Source: CAD feature listing. Evaluate the final solid. Frame: model axes, mm. A direction names the side the tool comes from. Give positions to 0.01 mm unless a question says otherwise; leave off trailing zeros. Write each loop counter-clockwise with the first axis right and the second up, starting at its lowest first coordinate (ties: lowest second). Pieces come first, ordered by that corner, then holes. Notation, with made-up numbers: (-19.5, 18.5) - (27.5, 18.5) arc R23 ccw to (27.5, 33.5) - close; hole circle Ø2 at (75, 6). An arc over 180 degrees is marked (long way). One line per question, with ' | ' between items. Start each with the question number.
(1) Pin query (flat end, axial travel): pin 1 (5 mm diameter, centred on x = 12, z = 20.5, fed in from +Y); pin 2 (2.5 mm diameter, centred on y = -16, z = 33, fed in from -X); pin 3 (10 mm diameter, centred on x = 0, y = 0, fed in from +Z); pin 4 (12 mm diameter, centred on x = 18, y = 1.5, fed in from +Z). Return the tip coordinate at first contact, or that it passes through.
(2) Draft query along Y for faces 5 (the cylindrical face through (27, -16, 21)), 6 (the cylindrical face through (6.5, 0.07, 2.96)), 7 (the flat face through (0, -14.5, 21)). Return one class per face: +Y half, -Y half, draft (parallel to the pull), parting line (faces both ways), or undercut.
(3) Access query for faces 1 (the flat face through (17.5, 0, 3)), 2 (the flat face through (-17.5, 0, 3)), 3 (the flat face through (-17.5, -16, 33)), 4 (the flat face through (17.5, -16, 33)). Directions: +Z, -Z, +X, -X, +Y, -Y. A direction counts if a zero-diameter tool reaches every point of the face in a straight line with its end or side. Return the directions, or none.
(4) Ray query, line 1 (X direction, y = -16.4, z = 21); line 2 (Y direction, x = 0, z = 1.75); line 3 (Y direction, x = 8, z = 4.1). Return the intervals inside material, ascending. Write a range as [from, to].
(5) Section B-B, the plane y = 0. Return loops of the section in (x, z), plus the area to 3 significant figures.
(6) Section D-D, the plane z = 5. Return loops of the section in (x, y), plus the area to 3 significant figures.
(7) Section A-A, the plane x = 0. Return loops of the section in (y, z).
(8) Section C-C, the plane z = 21. Return loops of the section in (x, y), plus the area to 3 significant figures.
```python
from build123d import *

# Parameters (mm, degrees)
SKETCH1_W           = 35
SKETCH1_H           = 35
SKETCH1_R           = 5.5
SKETCH1_R_2         = 1.5
BOSS_EXTRUDE1_DEPTH = 6
SKETCH2_W           = 35
SKETCH2_H           = 3
BOSS_EXTRUDE2_DEPTH = 30
SKETCH3_R           = 1.5
BOSS_EXTRUDE3_DEPTH = 3


with BuildPart() as part:
    # Sketch1 → Boss-Extrude1 (new body)
    with BuildSketch(Plane.XY):
        Rectangle(SKETCH1_W, SKETCH1_H)
        Circle(SKETCH1_R, mode=Mode.SUBTRACT)
        with Locations((8, 0)):
            Circle(SKETCH1_R_2, mode=Mode.SUBTRACT)
        with Locations((-8, 0)):
            Circle(SKETCH1_R_2, mode=Mode.SUBTRACT)
    extrude(amount=BOSS_EXTRUDE1_DEPTH)

    # Sketch2 → Boss-Extrude2 (add)
    with BuildSketch(Plane.XY.offset(6)):
        with Locations((0, -16)):
            Rectangle(SKETCH2_W, SKETCH2_H)
    extrude(amount=BOSS_EXTRUDE2_DEPTH)

    # Sketch3 → Boss-Extrude3 (add)
    # profile 1 of 2: a face of its own
    with BuildSketch(Plane(origin=(0, -14.5, 0), x_dir=(1, 0, 0), z_dir=(0, 1, 0))):
        with BuildLine():
            Line((17.5, -29.75), (17.5, -12.25))
            Line((17.5, -12.25), (26.114080353, -19.090878575))
            ThreePointArc((26.114080353, -19.090878575), (27, -21), (26.114080353, -22.909121425))
            Line((26.114080353, -22.909121425), (17.5, -29.75))
        make_face()
        with Locations(Location((24.5, -21, 0), (0, 0, 270))):
            Circle(SKETCH3_R, mode=Mode.SUBTRACT)
    # profile 2 of 2: a face of its own
    with BuildSketch(Plane(origin=(0, -14.5, 0), x_dir=(1, 0, 0), z_dir=(0, 1, 0))):
        with BuildLine():
            Line((-17.5, -29.75), (-17.5, -12.25))
            Line((-17.5, -12.25), (-26.114080353, -19.090878575))
            ThreePointArc((-26.114080353, -19.090878575), (-27, -21), (-26.114080353, -22.909121425))
            Line((-26.114080353, -22.909121425), (-17.5, -29.75))
        make_face()
        with Locations(Location((-24.5, -21, 0), (0, 0, 270))):
            Circle(SKETCH3_R, mode=Mode.SUBTRACT)
    extrude(amount=-BOSS_EXTRUDE3_DEPTH)


solid = part.part
```
Check sheet entries:
1) pin 1: y = -14.5 | pin 2: x = -17.5 | pin 3: through | pin 4: z = 6
2) face 5: draft | face 6: undercut | face 7: +Y half
3) face 1: -Z, +X, +Y, -Y | face 2: -Z, -X, +Y, -Y | face 3: +Z, -X, +Y, -Y | face 4: +Z, +X, +Y, -Y
4) line 1: [-27, -26], [-23, 23], [26, 27] | line 2: [-17.5, -5.5], [5.5, 17.5] | line 3: [-17.5, -1.5], [1.5, 17.5]
5) outline: (-17.5, 0) - (-9.5, 0) - (-9.5, 6) - (-17.5, 6) - close; (-6.5, 0) - (-5.5, 0) - (-5.5, 6) - (-6.5, 6) - close; (5.5, 0) - (6.5, 0) - (6.5, 6) - (5.5, 6) - close; (9.5, 0) - (17.5, 0) - (17.5, 6) - (9.5, 6) - close | area: 108 mm²
6) outline: (-17.5, -17.5) - (17.5, -17.5) - (17.5, 17.5) - (-17.5, 17.5) - close; hole circle Ø3 at (-8, 0); hole circle Ø11 at (0, 0); hole circle Ø3 at (8, 0) | area: 1,120 mm²
7) outline: (-17.5, 0) - (-5.5, 0) - (-5.5, 6) - (-14.5, 6) - (-14.5, 36) - (-17.5, 36) - close; (5.5, 0) - (17.5, 0) - (17.5, 6) - (5.5, 6) - close
8) outline: (-27, -17.5) - (-26, -17.5) - (-26, -14.5) - (-27, -14.5) - close; (-23, -17.5) - (23, -17.5) - (23, -14.5) - (-23, -14.5) - close; (26, -17.5) - (27, -17.5) - (27, -14.5) - (26, -14.5) - close | area: 144 mm²
